Geometry: final body of the model. Coordinates: model frame, mm. Face numbers are marked on the shaded views. A direction names the side the tool comes from. Give positions to 0.01 mm unless a question says otherwise; leave off trailing zeros. Write each loop counter-clockwise with the first axis right and the second up, starting at its lowest first coordinate (ties: lowest second). Pieces come first, ordered by that corner, then holes.
Q1. Pin query (flat end, axial travel): pin 1 (1.5 mm diameter, centred on x = -1.5, z = 8, fed in from -Y); pin 2 (1 mm diameter, centred on y = -0.5, z = 14, fed in from -X); pin 3 (1 mm diameter, centred on x = -1.5, y = -1.5, fed in from -Z). Return the tip coordinate at first contact, or that it passes through.
Q2. Cut plane A-A on z = 7. Return the cut outline in (x, y).
Q3. Line query: L1, parallel to X at y = 0.35, z = 6.25; L2, parallel to Z at x = -1, y = -0.1. Output: solid intervals per line, ascending.
Q4. Reachability of the marked faces 1 and 2 from +Z, -Z, +X, -X, +Y, -Y: full face, straight path, thin tool, end or side. Return the list, or none.
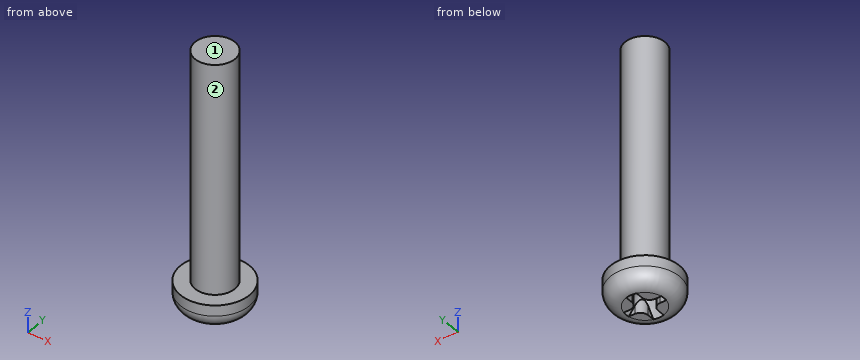
Autodesk Inventor part; units mm, degrees
ref_plane "YZ Plane" through (0, 0, 0) normal (1, 0, 0) x (0, 1, 0)
ref_plane "XZ Plane" through (0, 0, 0) normal (0, 1, 0) x (-1, 0, 0)
ref_plane "XY Plane" through (0, 0, 0) normal (0, 0, 1) x (1, 0, 0)
sketch "スケッチ1" plane through (0, 0, 0) normal (1, 0, 0) x (0, 1, 0)
  line L0 (0, 16.7) -> (0, 0)
  line L1 (0, 0) -> (1.25, 0)
  line L2 (2.25, 1) -> (2.25, 1.7)
  line L3 (2.25, 1.7) -> (1.3, 1.7)
  line L4 (1.3, 1.7) -> (1.3, 16.7)
  line L5 (1.3, 16.7) -> (0, 16.7)
  line L6 (1.25, 0) -> (0, 1.7)
  arc A0 (1.25, 0) -> (2.25, 1) centre (1.25, 1) ccw
  line L7 (1.25, 0) -> (2.25, 0)
  line L8 (2.25, 0) -> (2.25, 1)
  dimension "d2" = 1.7
  dimension "d10" = 15
  dimension "d11" = 2.6
  dimension "d12" = 4.5
  dimension "d14" = 1
revolve "回転1" add sketch "スケッチ1" angle 360 about axis through (0, 0, 16.7) along (0, 0, -1) contours L5 L4 L3 L2 A0 L6 L0
thread "ねじ1"
sketch "スケッチ2" plane through (0, 0, 1.7) normal (0, 0, 1) x (1, 0, 0)
  line L0 (0.3339, -1.6357) -> (-0.3339, -1.6357)
  line L1 (-0.3339, -1.6357) -> (-0.3339, -0.7226)
  line L2 (-0.3339, 1.6357) -> (0.3339, 1.6357)
  line L3 (0.3339, 1.6357) -> (0.3339, 0.7226)
  line L4 (0.3339, -1.6357) -> (-0.3339, 1.6357) construction
  line L5 (-0.3339, -1.6357) -> (0.3339, 1.6357) construction
  line L6 (-1.5922, 0.2226) -> (-0.8339, 0.2226)
  line L7 (1.5922, 0.2226) -> (1.5922, -0.2226)
  line L8 (1.5922, -0.2226) -> (0.8339, -0.2226)
  line L9 (-1.5922, -0.2226) -> (-1.5922, 0.2226)
  line L10 (-1.5922, 0.2226) -> (1.5922, -0.2226) construction
  line L11 (1.5922, 0.2226) -> (-1.5922, -0.2226) construction
  circle A0 centre (0, 0) radius 2.25
  line L12 (0.3339, -0.7226) -> (0.3339, -1.6357)
  line L13 (0.8339, 0.2226) -> (1.5922, 0.2226)
  line L14 (-0.8339, -0.2226) -> (-1.5922, -0.2226)
  line L15 (-0.3339, 0.7226) -> (-0.3339, 1.6357)
  arc A1 (0.8339, -0.2226) -> (0.3339, -0.7226) centre (0.8339, -0.7226) ccw
  arc A2 (0.3339, 0.7226) -> (0.8339, 0.2226) centre (0.8339, 0.7226) ccw
  arc A3 (-0.8339, 0.2226) -> (-0.3339, 0.7226) centre (-0.8339, 0.7226) ccw
  arc A4 (-0.3339, -0.7226) -> (-0.8339, -0.2226) centre (-0.8339, -0.7226) ccw
  point P0 (-0.3339, -0.2226)
  point P1 (-0.3339, 0.2226)
  point P2 (0.3339, 0.2226)
  point P3 (0.3339, -0.2226)
  dimension "d18" = 0.5
extrude "押し出し2" add sketch "スケッチ2" against normal blind 1.7
revolve "回転2" cut sketch "スケッチ1" angle 360 about axis through (0, 0, 16.7) along (0, 0, -1) contours A0 L8 L7
properties part number "F-2615EB" material "チタン"
Data:
1. pin 1: stops at y = -1.06
1. pin 2: stops at x = -1.3
1. pin 3: stops at z = 0.07
2. outline: circle Ø2.6 at (0, 0)
3. L1: x = -1.25 to 1.25
3. L2: z = 0.33 to 16.7
4. face 1: +Z, +X, -X, +Y, -Y
4. face 2: +Z
